Could you check a few things on this model? Use its own coordinates, in mm. A direction names the side the tool comes from. Round coordinates to 2 decimals unless told otherwise and drop trailing zeros. Loops run counter-clockwise (first coordinate to the right, second up) from the corner with the lowest first, then second, coordinate; pieces in that order, holes last. Notation, with made-up numbers: (80, 43.25) -> (115, 43.25) arc R30 ccw to (115, 70.25) -> close; hole circle Ø8 at (-4, 32). An arc over 180 degrees is marked (long way). One line per item, written item: value.
Autodesk Inventor part; units mm, degrees
ref_plane "YZ Plane" through (0, 0, 0) normal (1, 0, 0) x (0, 1, 0)
ref_plane "XZ Plane" through (0, 0, 0) normal (0, 1, 0) x (-1, 0, 0)
sketch "Sketch1" plane through (0, 0, 0) normal (0, 1, 0) x (-1, 0, 0)
  circle A0 centre (0, 0) radius 4.7674
  circle A1 centre (0, 0) radius 10
  line L0 (9.8737, 1.5843) -> (9.8737, -1.5843)
  line L1 (9.8737, -1.5843) -> (12.5697, -1.5843)
  line L2 (12.5697, -1.5843) -> (12.5697, 1.5843)
  line L3 (12.5697, 1.5843) -> (9.8737, 1.5843)
  dimension "d0" = 20
  dimension "d1" = 9.5349
extrude "Extrusion1" add sketch "Sketch1" along normal blind 10
properties part number "Test_gear_p1"
Item 1: I need wall thicknesses on line 1 (Z direction, x = 0.25, y = 6.25); line 2 (X direction, y = 3, z = -3); line 3 (Z direction, x = -4.25, y = 2.25). Which ranges of each line are inside material? Lowest first, please. Write a range as from..to.
Output:
line 1: z = -10..-4.76, 4.76..10
line 2: x = -9.54..-3.71, 3.71..9.54
line 3: z = -9.05..-2.16, 2.16..9.05
Item 2: If we section it at C-C on y = 5.5: List the corners of the cut face in (x, z) for me, plus the area to 3 significant figures.
Output:
outline: (-12.57, -1.58) -> (-9.87, -1.58) arc R10 ccw (long way) to (-9.87, 1.58) -> (-12.57, 1.58) -> close; hole circle Ø9.53 at (0, 0)
area: 251 mm²
Item 3: For faces 4 (the face through (10, 5, 0)), 5 (the face through (-11, 5, -1.584)), which set-ups out of +Z, -Z, +X, -X, +Y, -Y let a thin tool reach every point of the face, with its end or its side?
Output:
face 4: +Y, -Y
face 5: -Z, -X, +Y, -Y
Item 4: Will these pins go through, and if not, where does the flat tip stop? pin 1 Ø1.5 at (y, z) = (5, 6.5) entering from +X; pin 2 Ø3 at (x, y) = (-12, 5) entering from -Z; pin 3 Ø4 at (y, z) = (4, 6) entering from -X.
Output:
pin 1: stops at x = 8.18
pin 2: stops at z = -1.58
pin 3: stops at x = -9.17
Item 5: If we mould it in two halves opening along Z, with no side actions, what happens to faces 1 (the face through (-11, 5, 1.584)), 2 (the face through (-2.2, 4.93, 4.23)), 3 (the face through (1, 0, 5))? For each: released by +Z, released by -Z, zero draft, split by the parting line, or undercut.
Output:
face 1: released by +Z
face 2: undercut
face 3: zero draft
Item 6: If we section it at B-B on z = 0: List the corners of the cut face in (x, y) for me.
Output:
outline: (-12.57, 0) -> (-4.77, 0) -> (-4.77, 10) -> (-12.57, 10) -> close; (4.77, 0) -> (10, 0) -> (10, 10) -> (4.77, 10) -> close
Item 7: If we section it at D-D on z = 8: List the corners of the cut face in (x, y) for me, plus the area to 3 significant figures.
Output:
outline: (-6, 0) -> (6, 0) -> (6, 10) -> (-6, 10) -> close
area: 120 mm²
Item 8: If we section it at A-A on x = 0: List the corners of the cut face in (y, z) for me.
Output:
outline: (0, -10) -> (10, -10) -> (10, -4.77) -> (0, -4.77) -> close; (0, 4.77) -> (10, 4.77) -> (10, 10) -> (0, 10) -> close
